For this review, take the finished solid that the model builds, in its own axes (mm). A direction names the side the tool comes from. Round coordinates to 2 decimals unless told otherwise and drop trailing zeros. Write each loop counter-clockwise with the first axis right and the second up, starting at its lowest first coordinate (ties: lowest second). Pieces come first, ordered by that corner, then holes. Notation, with made-up numbers: (47, 2) -> (93, 2) arc R11 ccw to (93, 21) -> close; hole circle Ø10 at (45, 62). An arc over 180 degrees is marked (long way). Answer in a Markdown table with one row per item. Add a question column.
```python
from build123d import *

# Parameters (mm, degrees)
SKETCH1_R               = 2.95
BOSS_EXTRUDE4_DEPTH     = 1
SKETCH2_R               = 2.5
BOSS_EXTRUDE5_DEPTH     = 7.8
SKETCH4_W               = 16.58699552
SKETCH4_H               = 3.788232685
CUT_EXTRUDE2_DEPTH      = 8.8
CUT_EXTRUDE2_DEPTH_BACK = 2


with BuildPart() as part:
    # Sketch1 → Boss-Extrude4 (new body)
    with BuildSketch(Plane(origin=(0, 0, 0), x_dir=(1, 0, 0), z_dir=(0, 1, 0))):
        Circle(SKETCH1_R)
    extrude(amount=BOSS_EXTRUDE4_DEPTH)

    # Sketch2 → Boss-Extrude5 (add)
    with BuildSketch(Plane(origin=(0, 1, 0), x_dir=(1, 0, 0), z_dir=(0, 1, 0))):
        Circle(SKETCH2_R)
    extrude(amount=BOSS_EXTRUDE5_DEPTH)

    # Sketch3 → Cut-Revolve5 (revolve, cut)
    with BuildSketch(Plane(origin=(0, 0, 0), x_dir=(0, 0, -1), z_dir=(1, 0, 0))):
        with BuildLine():
            ThreePointArc((0, 8.8), (-1.767766953, 8.067766953), (-2.5, 6.3))
            Line((-2.5, 6.3), (-2.5, 1))
            Line((-2.5, 1), (-5.449902287, 1))
            Line((-5.449902287, 1), (-5.449902287, 10.727798838))
            Line((-5.449902287, 10.727798838), (0, 10.727798838))
            Line((0, 10.727798838), (0, 8.8))
        make_face()
    revolve(axis=Axis((0, 11.133122405, 0), (0, -1, 0)), mode=Mode.SUBTRACT)

    # Sketch4 → Cut-Extrude2 (cut, two sides)
    with BuildSketch(Plane(origin=(0, 1, 0), x_dir=(1, 0, 0), z_dir=(0, 1, 0))) as cut_extrude2_sk:
        with Locations((1.563846093, -4.394116343)):
            Rectangle(SKETCH4_W, SKETCH4_H)
    extrude(amount=CUT_EXTRUDE2_DEPTH, mode=Mode.SUBTRACT)
    extrude(cut_extrude2_sk.sketch, amount=-CUT_EXTRUDE2_DEPTH_BACK, mode=Mode.SUBTRACT)


solid = part.part
```
1. We need section B-B (x = -0.5). Write out the cut boundary in (y, z), plus the area to 3 significant figures.
2. For L1, parallel to Y at x = 1.6, z = 2.15; L2, parallel to Y at x = -1.3, z = 0.5; L3, parallel to Z at x = 1.1, y = 7, list the stretches that pass through material, from the lowest coordinate up. Write a range as [from, to].
3. We need section C-C (y = 1.75). Write out the cut boundary in (x, z).
4. Clearance check with flat-ended pins moving along their axes: pin 1 Ø1.5 at (x, z) = (0, -1.5) entering from +Y; pin 2 Ø3 at (x, z) = (2, -1.5) entering from +Y. State where each tip first meets the part, or that it passes through.
5. We need section A-A (z = 0). Write out the cut boundary in (x, y).
6. We need section D-D (y = 7). Write out the cut boundary in (x, z), plus the area to 3 significant figures.
7. Tool access review of faces 1 (the cylindrical face through (-0.54, 3.61, 2.44)), 2 (the flat face through (0, 0.5, 2.5)): name each direction out of +Z, -Z, +X, -X, +Y, -Y from which nothing blocks a thin tool from reaching the whole face with its end or side.
Response:
| question | item | result |
|---|---|---|
| 1 | outline | (0, -2.91) -> (1, -2.91) -> (1, -2.45) -> (6.3, -2.45) arc R2.45 ccw to (6.3, 2.45) -> (1, 2.45) -> (1, 2.5) -> (0, 2.5) -> close |
| 1 | area | 40.8 mm2 |
| 2 | L1 | [0, 1] |
| 2 | L2 | [0, 8.38] |
| 2 | L3 | [-2.13, 2.13] |
| 3 | outline | circle Ø5 at (0, 0) |
| 4 | pin 1 | y = 8.68 |
| 4 | pin 2 | y = 8.59 |
| 5 | outline | (-2.95, 0) -> (2.95, 0) -> (2.95, 1) -> (2.5, 1) -> (2.5, 6.3) arc R2.5 ccw to (-2.5, 6.3) -> (-2.5, 1) -> (-2.95, 1) -> close |
| 6 | outline | circle Ø4.8 at (0, 0) |
| 6 | area | 18.1 mm2 |
| 7 | face 1 | +Y |
| 7 | face 2 | +Z, +X, -X, +Y, -Y |
